```python
from build123d import *

# Parameters (mm, degrees)
SKETCH2_R                    = 50.8
BOSS_EXTRUDE1_DEPTH          = 25.4
FILLET1_R                    = 2.54
BOSS_EXTRUDE2_START          = -25.4
BOSS_EXTRUDE2_DEPTH          = 5.08
CHAMFER1_SIZE                = 3.81
BOSS_EXTRUDE3_DEPTH          = 2.54
BOSS_EXTRUDE4_DEPTH          = 1.27
BOSS_EXTRUDE6_DEPTH          = 2.54
BOSS_EXTRUDE7_DEPTH          = 1.27
CIRPATTERN1_COUNT            = 4
CHAMFER1_OF_CIRPATTERN1_SIZE = 3.81
CIRPATTERN2_COUNT            = 4
SKETCH12_R                   = 38.1
BOSS_EXTRUDE8_DEPTH          = 2.54
FILLET2_R                    = 2.54
SKETCH13_R                   = 6.35
BOSS_EXTRUDE9_DEPTH          = 5.08


with BuildPart() as part:
    # Sketch2 → Boss-Extrude1 (new body)
    with BuildSketch(Plane(origin=(0, 0, 0), x_dir=(1, 0, 0), z_dir=(0, 1, 0))):
        with Locations(Location((-3.216165312, 3.339863978, 0), (0, 0, 270))):
            Circle(SKETCH2_R)
    extrude(amount=BOSS_EXTRUDE1_DEPTH)

    # Fillet1
    fillet1_edges = [part.edges().sort_by_distance(p)[0] for p in [
        (-3.216165312, 25.4, -54.139863978),
    ]]
    fillet(fillet1_edges, radius=FILLET1_R)

    # Sketch3 → Boss-Extrude2 (add)
    with BuildSketch(Plane(origin=(0, 25.4, 0), x_dir=(1, 0, 0), z_dir=(0, 1, 0)).offset(BOSS_EXTRUDE2_START)):
        with BuildLine():
            Line((-53.115207137, 12.864863978), (-65.815207137, 12.864863978))
            Line((-65.815207137, 12.864863978), (-65.815207137, -6.185136022))
            Line((-65.815207137, -6.185136022), (-53.115207137, -6.185136022))
            ThreePointArc((-53.115207137, -6.185136022), (-54.016165312, 3.339863978), (-53.115207137, 12.864863978))
        make_face()
    boss_extrude2 = extrude(amount=BOSS_EXTRUDE2_DEPTH)

    # Chamfer1
    chamfer1_edges = [part.edges().sort_by_distance(p)[0] for p in [
        (-65.815207137, 2.54, -12.864863978),
        (-65.815207137, 2.54, 6.185136022),
    ]]
    chamfer(chamfer1_edges, length=CHAMFER1_SIZE)

    # Sketch4 → Boss-Extrude3 (add)
    with BuildSketch(Plane.XY.offset(6.185136022)):
        Polygon((-53.115207137, 5.08), (-53.115207137, 22.86), (-58.195207137, 22.86), (-62.005207137, 5.08), align=None)
    boss_extrude3 = extrude(amount=-BOSS_EXTRUDE3_DEPTH)

    # Sketch5 → Boss-Extrude4 (add)
    with BuildSketch(Plane(origin=(0, 5.08, 0), x_dir=(1, 0, 0), z_dir=(0, 1, 0))):
        Polygon((-63.654985531, -0.787636022), (-62.005207137, -1.740136022), (-60.355428742, -0.787636022), (-60.355428742, 1.117363978), (-62.005207137, 2.069863978), (-63.654985531, 1.117363978), align=None)
    boss_extrude4 = extrude(amount=BOSS_EXTRUDE4_DEPTH)

    # Sketch10 → Boss-Extrude6 (add)
    with BuildSketch(Plane(origin=(0, 0, -12.864863978), x_dir=(-1, 0, 0), z_dir=(0, 0, -1))):
        Polygon((53.115207137, 5.08), (53.115207137, 22.86), (57.19920047, 22.86), (62.005207137, 5.08), align=None)
    boss_extrude6 = extrude(amount=-BOSS_EXTRUDE6_DEPTH)

    # Sketch11 → Boss-Extrude7 (add)
    with BuildSketch(Plane(origin=(0, 5.08, 0), x_dir=(1, 0, 0), z_dir=(0, 1, 0))):
        Polygon((-63.745716673, 6.046159142), (-62.005207137, 5.041275493), (-60.264697601, 6.046159142), (-60.264697601, 8.05592644), (-62.005207137, 9.060810089), (-63.745716673, 8.05592644), align=None)
    boss_extrude7 = extrude(amount=BOSS_EXTRUDE7_DEPTH)

    # CirPattern1: Boss-Extrude2, Boss-Extrude3, Boss-Extrude6 ×4 about axis
    cirpattern1_axis = Axis((-3.216165312, 0, -3.339863978), (0, 1, 0))
    add([boss_extrude2.rotate(cirpattern1_axis, i * 360 / CIRPATTERN1_COUNT) for i in range(1, CIRPATTERN1_COUNT)])
    add([boss_extrude3.rotate(cirpattern1_axis, i * 360 / CIRPATTERN1_COUNT) for i in range(1, CIRPATTERN1_COUNT)])
    add([boss_extrude6.rotate(cirpattern1_axis, i * 360 / CIRPATTERN1_COUNT) for i in range(1, CIRPATTERN1_COUNT)])

    # Chamfer1 of CirPattern1
    chamfer1_of_cirpattern1_edges = [part.edges().sort_by_distance(p)[0] for p in [
        (-12.741165312, 2.54, 59.259177846),
        (6.308834688, 2.54, 59.259177846),
        (59.382876512, 2.54, 6.185136022),
        (59.382876512, 2.54, -12.864863978),
        (6.308834688, 2.54, -65.938905803),
        (-12.741165312, 2.54, -65.938905803),
    ]]
    chamfer(chamfer1_of_cirpattern1_edges, length=CHAMFER1_OF_CIRPATTERN1_SIZE)

    # CirPattern2: Boss-Extrude4, Boss-Extrude7 ×4 about axis
    cirpattern2_axis = Axis((-3.216165312, 0, -3.339863978), (0, 1, 0))
    add([boss_extrude4.rotate(cirpattern2_axis, i * 360 / CIRPATTERN2_COUNT) for i in range(1, CIRPATTERN2_COUNT)])
    add([boss_extrude7.rotate(cirpattern2_axis, i * 360 / CIRPATTERN2_COUNT) for i in range(1, CIRPATTERN2_COUNT)])

    # Sketch12 → Boss-Extrude8 (add)
    with BuildSketch(Plane(origin=(0, 25.4, 0), x_dir=(1, 0, 0), z_dir=(0, 1, 0))):
        with Locations(Location((-3.216165312, 3.339863978, 0), (0, 0, 270))):
            Circle(SKETCH12_R)
    extrude(amount=BOSS_EXTRUDE8_DEPTH)

    # Fillet2
    fillet2_edges = [part.edges().sort_by_distance(p)[0] for p in [
        (-3.216165312, 27.94, -41.439863978),
    ]]
    fillet(fillet2_edges, radius=FILLET2_R - 0.0001)  # a hair under: the kernel refuses the full size

    # Sketch13 → Boss-Extrude9 (add)
    with BuildSketch(Plane(origin=(0, 27.94, 0), x_dir=(1, 0, 0), z_dir=(0, 1, 0))):
        with Locations(Location((-3.216165312, 3.339863978, 0), (0, 0, 270))):
            Circle(SKETCH13_R)
    extrude(amount=BOSS_EXTRUDE9_DEPTH)


solid = part.part
```
Verification items for the finished model (mm, model axes). A direction names the side the tool comes from. Give positions to 0.01 mm unless a question says otherwise; leave off trailing zeros. Write each loop counter-clockwise with the first axis right and the second up, starting at its lowest first coordinate (ties: lowest second). Pieces come first, ordered by that corner, then holes. Notation, with made-up numbers: (14, -16.75) - (70, -16.75) arc R18 ccw to (70, -7.75) - close; hole circle Ø2 at (-17.5, 12.5). An arc over 180 degrees is marked (long way). Put each result on its own line as item: value.
Q1. Scan lines: probe 1 along Y at (x, z) = (15.5, 35); probe 2 along Y at (x, z) = (-36, -10.5); probe 3 along X at (y, z) = (7.5, -3). Record each from-to range of solid material in increasing order. Write a range as from..to.
Result:
probe 1: 0..25.4
probe 2: 0..27.94
probe 3: -54.02..47.58
Q2. Set-up check for faces 1 (the face through (-10.201, 12, 50)), 2 (the face through (-11.489, 14.094, 53.013)), 3 (the face through (-57, 9, -12.865)): record each of +Z, -Z, +X, -X, +Y, -Y from which the full face is reachable in a straight line by a thin tool's end or side.
Result:
face 1: +Z, +Y
face 2: +Z, -X, +Y
face 3: -Z, -X, +Y, -Y
Q3. Section check A-A on y = 3.5. Record the cut outline in (x, z), and give its area (3 significant figures).
Result:
outline: (-65.82, -9.05) - (-62.01, -12.86) - (-53.12, -12.86) arc R50.8 ccw to (-12.74, -53.24) - (-12.74, -62.13) - (-8.93, -65.94) - (2.5, -65.94) - (6.31, -62.13) - (6.31, -53.24) arc R50.8 ccw to (46.68, -12.86) - (55.57, -12.86) - (59.38, -9.05) - (59.38, 2.38) - (55.57, 6.19) - (46.68, 6.19) arc R50.8 ccw to (6.31, 46.56) - (6.31, 55.45) - (2.5, 59.26) - (-8.93, 59.26) - (-12.74, 55.45) - (-12.74, 46.56) arc R50.8 ccw to (-53.12, 6.19) - (-62.01, 6.19) - (-65.82, 2.38) - close
area: 8,970 mm2
Q4. Section check C-C on y = 29.5. Record the cut outline in (x, z).
Result:
outline: circle Ø12.7 at (-3.22, -3.34)
Q5. Depth check by flat-ended pin: P1, Ø10, axis at y = 10, z = -59, coming from the -X side; P2, Ø1, axis at y = 6, z = 0, coming from the +X side; P3, Ø3, axis at y = 11.5, z = 15, coming from the -X side; P4, Ø3, axis at x = -40, y = 29.5, coming from the -Z side. Enter the tip coordinate at first touch or a pass-through.
Result:
P1: x = -12.74
P2: x = 57.31
P3: x = -51.14
P4: through
Q6. Mould release check, pull along Z, two halves, no side actions. Record for faces 4 (the face through (53, 5.08, -3)), 5 (the face through (-7, 6.35, 55)), 6 (the face through (-3, 5.08, 53)), 7 (the face through (5.057, 14.094, -59.692)): released by +Z, released by -Z, zero draft, split by the parting line, or undercut.
Result:
face 4: undercut
face 5: zero draft
face 6: undercut
face 7: released by -Z
